For this review, use the dimensioned drawing (mm, ordinates from the lowest corner) and the shaded views. A direction names the side the tool comes from. Coordinates: 2 decimals unless noted, no trailing zeros. Loops run counter-clockwise (first coordinate to the right, second up) from the corner with the lowest first, then second, coordinate; pieces in that order, holes last.
1. To check wall thickness, follow probe 1 along X at (y, z) = (72.5, 8.5); probe 2 along Y at (x, z) = (75.5, 6); probe 3 along Z at (x, y) = (47, 65.5). State the ranges of each line that lie inside material, in increasing order.
2. Clearance check with flat-ended pins moving along their axes: P1, Ø0.9, axis at x = 104, y = 115, coming from the -Z side; P2, Ø8, axis at x = 13.83, y = 16.72, coming from the +Z side; P3, Ø16, axis at x = 92.17, y = 16.72, coming from the -Z side. State where each tip first meets the part, or that it passes through.
3. Mouldability with a two-part tool opening along Y and no side actions: class the marked faces 3, 4 and 5 as pulls with the +Y half, pulls with the -Y half, needs draft (parallel to the pull), parting line crosses it, or undercut.
4. Machinability: for the marked faces 1 and 2, which of the approach directions +Z, -Z, +X, -X, +Y, -Y give a long, thin tool a straight path to every point of the face, cutting with its end or side? Answer none if there is none.
5. Take a section at A-A, the plane z = 4.5. State the section outline as (x, y) points, then the cut area to 3 significant figures.
6. Take a section at D-D, the plane y = 186.5. State the section outline as (x, z) points, then the cut area to 3 significant figures.
7. Take a section at C-C, the plane y = 143. State the section outline as (x, z) points.
8. Take a section at B-B, the plane x = 12. State the section outline as (y, z) points, then the cut area to 3 significant figures.
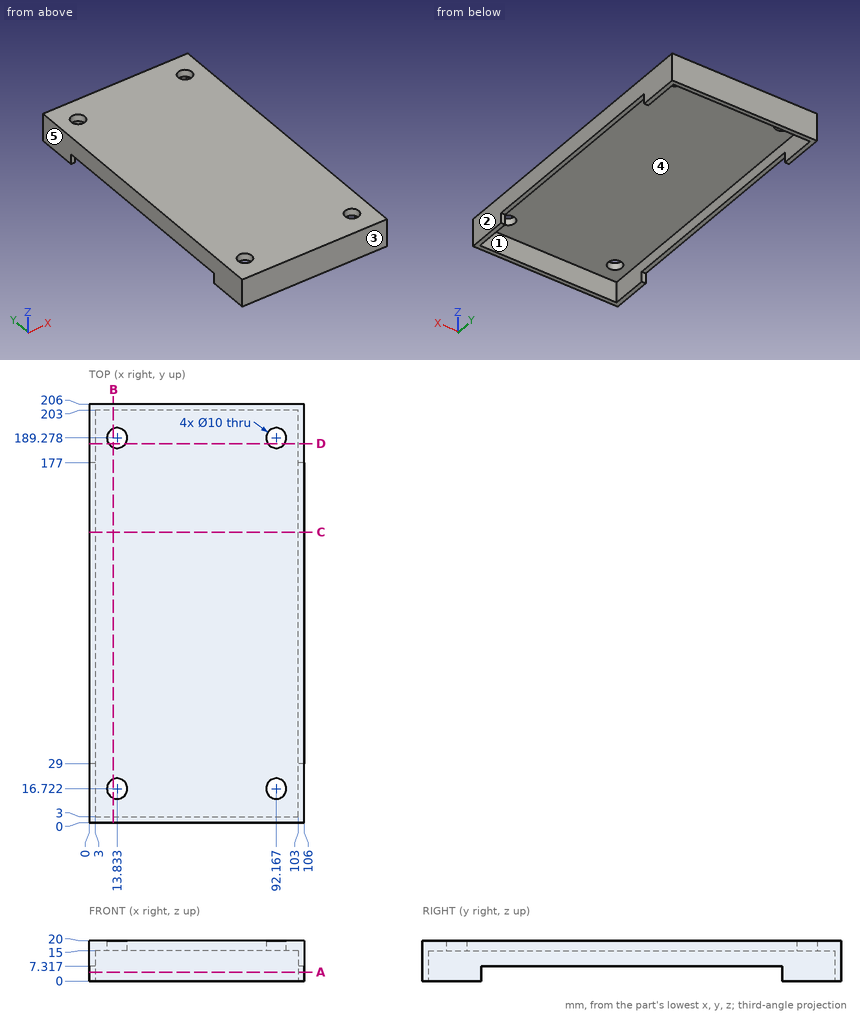
Results list:
1. probe 1: x = 0 to 3, 103 to 106
1. probe 2: y = 0 to 3, 203 to 206
1. probe 3: z = 15 to 20
2. P1: stops at z = 7.32
2. P2: passes through
2. P3: stops at z = 15
3. face 3: pulls with the -Y half
3. face 4: undercut
3. face 5: needs draft
4. face 1: -Z
4. face 2: +Z, -Z, +X, +Y, -Y
5. outline: (0, 0) - (106, 0) - (106, 29) - (103, 29) - (103, 3) - (3, 3) - (3, 29) - (0, 29) - close; (0, 177) - (3, 177) - (3, 203) - (103, 203) - (103, 177) - (106, 177) - (106, 206) - (0, 206) - close
5. area: 948 mm2
6. outline: (0, 0) - (3, 0) - (3, 15) - (9.68, 15) - (9.68, 20) - (0, 20) - close; (17.99, 15) - (88.01, 15) - (88.01, 20) - (17.99, 20) - close; (96.32, 15) - (103, 15) - (103, 0) - (106, 0) - (106, 20) - (96.32, 20) - close
6. area: 537 mm2
7. outline: (0, 7.32) - (3, 7.32) - (3, 15) - (103, 15) - (103, 7.32) - (106, 7.32) - (106, 20) - (0, 20) - close
8. outline: (0, 0) - (3, 0) - (3, 15) - (12.07, 15) - (12.07, 20) - (0, 20) - close; (21.37, 15) - (184.63, 15) - (184.63, 20) - (21.37, 20) - close; (193.93, 15) - (203, 15) - (203, 0) - (206, 0) - (206, 20) - (193.93, 20) - close
8. area: 1,030 mm2
